Check sheet for the modelled part. Datum: model origin and axes. Units: mm. Round coordinates to 2 decimals unless told otherwise and drop trailing zeros. Loops run counter-clockwise (first coordinate to the right, second up) from the corner with the lowest first, then second, coordinate; pieces in that order, holes last. Notation, with made-up numbers: (50, 85.5) -> (87, 85.5) arc R10 cw to (87, 94.5) -> close; hole circle Ø1 at (-30, 18.25). An arc over 180 degrees is marked (long way). One line per question, with ' | ' between items.
```python
from build123d import *

# Parameters (mm, degrees)
SKETCH1_R          = 4
SKETCH1_R_2        = 1.5
EXTRUDE_1319_DEPTH = 2
SKETCH3_R          = 5
EXTRUDE3_DEPTH     = 70.455021417


with BuildPart() as part:
    # Sketch1 → Extrude 1319 (new body)
    with BuildSketch(Plane.XY):
        with BuildLine():
            Line((59.5, -14), (68, -14))
            Line((68, -14), (68, 14))
            Line((68, 14), (59.5, 14))
            Line((59.5, 14), (-0.667028635, 9.97772884))
            ThreePointArc((-0.667028635, 9.97772884), (-10, 0), (-0.667028635, -9.97772884))
            Line((-0.667028635, -9.97772884), (59.5, -14))
        make_face()
        Circle(SKETCH1_R, mode=Mode.SUBTRACT)
        with Locations((7, 0)):
            Circle(SKETCH1_R_2, mode=Mode.SUBTRACT)
        with Locations((0, -7)):
            Circle(SKETCH1_R_2, mode=Mode.SUBTRACT)
        with Locations((-7, 0)):
            Circle(SKETCH1_R_2, mode=Mode.SUBTRACT)
        with Locations((0, 7)):
            Circle(SKETCH1_R_2, mode=Mode.SUBTRACT)
        with Locations((63.75, -9)):
            Circle(SKETCH1_R_2, mode=Mode.SUBTRACT)
        with Locations((63.75, 9)):
            Circle(SKETCH1_R_2, mode=Mode.SUBTRACT)
    extrude(amount=EXTRUDE_1319_DEPTH)

    # Sketch3 → Extrude3 (cut, through all)
    with BuildSketch(Plane(origin=(0, 0, 0), x_dir=(-1, 0, 0), z_dir=(0, 0, -1))):
        with Locations((-45, 0)):
            Circle(SKETCH3_R)
        with BuildLine():
            Line((-27, -2.5), (-23, -2.5))
            ThreePointArc((-23, -2.5), (-22, -3.5), (-23, -4.5))
            Line((-23, -4.5), (-27, -4.5))
            ThreePointArc((-27, -4.5), (-28, -3.5), (-27, -2.5))
        make_face()
        with BuildLine():
            Line((-27, 2.5), (-23, 2.5))
            ThreePointArc((-23, 2.5), (-22, 3.5), (-23, 4.5))
            Line((-23, 4.5), (-27, 4.5))
            ThreePointArc((-27, 4.5), (-28, 3.5), (-27, 2.5))
        make_face()
    extrude(amount=-EXTRUDE3_DEPTH, mode=Mode.SUBTRACT)


solid = part.part
```
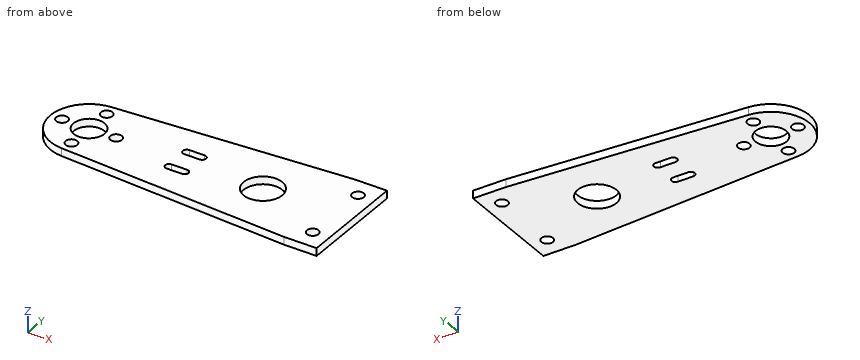
(1) Sectioned sample at B-B, the plane y = 0. Record the cut outline in (x, z).
Answer:
outline: (-10, 0) -> (-8.5, 0) -> (-8.5, 2) -> (-10, 2) -> close; (-5.5, 0) -> (-4, 0) -> (-4, 2) -> (-5.5, 2) -> close; (4, 0) -> (5.5, 0) -> (5.5, 2) -> (4, 2) -> close; (8.5, 0) -> (40, 0) -> (40, 2) -> (8.5, 2) -> close; (50, 0) -> (68, 0) -> (68, 2) -> (50, 2) -> close
(2) Go/stop test with flat-tipped pins: pin 1 (16 mm diameter, centred on x = 45, y = 0, fed in from -Z); pin 2 (0.6 mm diameter, centred on x = 24.5, z = 1, fed in from -Y); pin 3 (1 mm diameter, centred on x = 45.5, z = 1.5, fed in from +Y). Record where each tip stops, or that it passes through.
Answer:
pin 1: stops at z = 0 | pin 2: stops at y = -11.68 | pin 3: stops at y = 13.1
(3) Sectioned sample at A-A, the plane x = 63.75. Record the cut outline in (y, z).
Answer:
outline: (-14, 0) -> (-10.5, 0) -> (-10.5, 2) -> (-14, 2) -> close; (-7.5, 0) -> (7.5, 0) -> (7.5, 2) -> (-7.5, 2) -> close; (10.5, 0) -> (14, 0) -> (14, 2) -> (10.5, 2) -> close
(4) Scan lines: probe 1 along Y at (x, z) = (0, 0.6); probe 2 along X at (y, z) = (2.25, 1.2); probe 3 along X at (y, z) = (2.75, 0.2). Record each from-to range of solid material in increasing order.
Answer:
probe 1: y = -10.02 to -8.5, -5.5 to -4, 4 to 5.5, 8.5 to 10.02 | probe 2: x = -9.74 to -3.31, 3.31 to 40.53, 49.47 to 68 | probe 3: x = -9.61 to -2.9, 2.9 to 22.34, 27.66 to 40.82, 49.18 to 68
(5) Sectioned sample at C-C, the plane y = 6.25. Record the cut outline in (x, z), and give its area (3 significant figures).
Answer:
outline: (-7.81, 0) -> (-1.3, 0) -> (-1.3, 2) -> (-7.81, 2) -> close; (1.3, 0) -> (68, 0) -> (68, 2) -> (1.3, 2) -> close | area: 146 mm2
(6) Sectioned sample at D-D, the plane x = 7. Record the cut outline in (y, z).
Answer:
outline: (-10.49, 0) -> (-1.5, 0) -> (-1.5, 2) -> (-10.49, 2) -> close; (1.5, 0) -> (10.49, 0) -> (10.49, 2) -> (1.5, 2) -> close
